For this review, use the dimensioned drawing (mm, ordinates from the lowest corner) and the shaded views. A direction names the side the tool comes from. Give positions to 0.01 mm unless a question says otherwise; leave off trailing zeros. Loops run counter-clockwise (first coordinate to the right, second up) from the corner with the lowest first, then second, coordinate; pieces in that order, holes last. Notation, with made-up numbers: (31, 52.5) -> (60, 52.5) arc R9 ccw to (60, 66.5) -> close; hole circle Ø11 at (-14, 12). An arc over 180 degrees is marked (long way). Write each question's results on one line, items separated by ' | '. Start each with the question number.
Q1. Machinability: for the marked faces 5 and 6, which of the approach directions +Z, -Z, +X, -X, +Y, -Y give a long, thin tool a straight path to every point of the face, cutting with its end or side? Answer none if there is none.
Q2. Insertion check: pin 1 Ø4 at (x, z) = (34.06, 8.38) entering from -Y; pin 2 Ø1.5 at (x, z) = (29.06, 8.38) entering from +Y. Each pin has a flat end and moves straight along its axis. Give the tip position at first contact, or say it passes through.
Q3. We need section B-B (y = 4.55). Write out the cut boundary in (x, z) (1 decimal).
Q4. Wall thickness on L1, parallel to X at y = 3.1, z = 6.5; L2, parallel to Z at x = 34, y = 2.15 (1 decimal); L3, parallel to X at y = 2.65, z = 9: over which ranges is each line inside the solid? List them lowest first. Write a range as [from, to].
Q5. Mouldability with a two-part tool opening along X and no side actions: class the marked faces 1, 2, 3 and 4 as released by +X, released by -X, zero draft, split by the parting line, or undercut.
Q6. We need section C-C (x = 9.5). Write out the cut boundary in (y, z) (1 decimal), plus the area to 3 significant figures.
Q7. We need section A-A (z = 10.5). Write out the cut boundary in (x, y), plus the area to 3 significant figures.
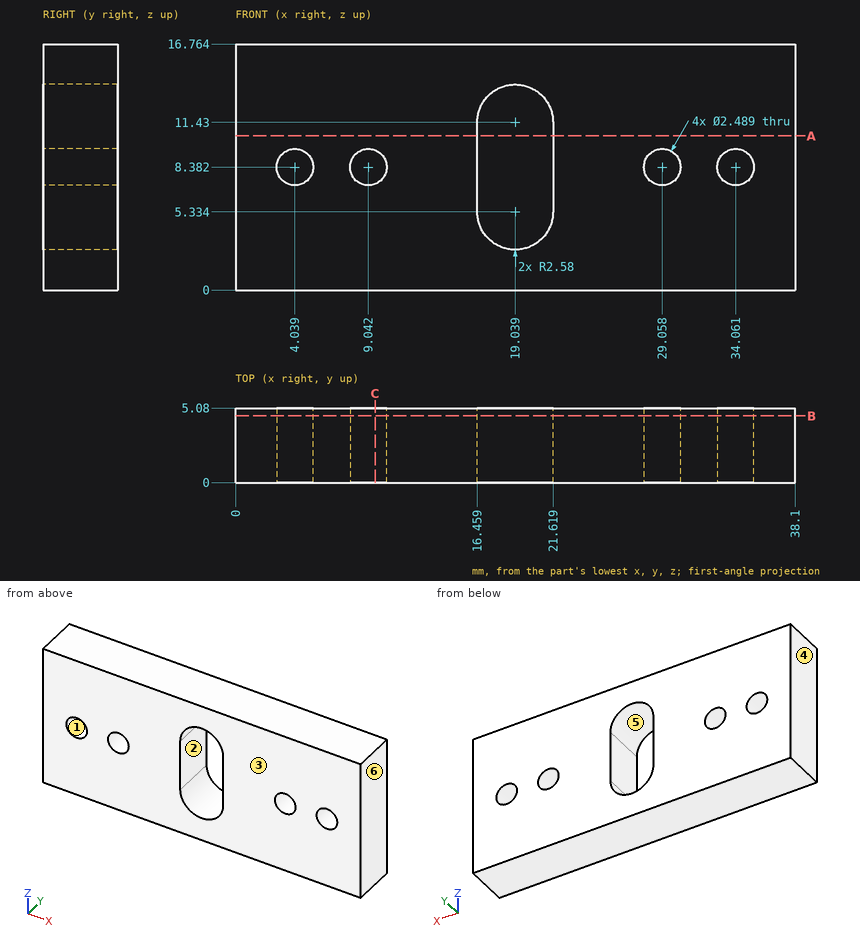
Output:
1) face 5: +Y, -Y | face 6: +Z, -Z, +X, +Y, -Y
2) pin 1: y = 0 | pin 2: through
3) outline: (0, 0) -> (38.1, 0) -> (38.1, 16.8) -> (0, 16.8) -> close; hole circle Ø2.5 at (4, 8.4); hole circle Ø2.5 at (9, 8.4); hole (16.5, 5.3) arc R2.6 ccw to (21.6, 5.3) -> (21.6, 11.4) arc R2.6 ccw to (16.5, 11.4) -> close; hole circle Ø2.5 at (29.1, 8.4); hole circle Ø2.5 at (34.1, 8.4)
4) L1: [0, 16.46], [21.62, 38.1] | L2: [0, 7.1], [9.6, 16.8] | L3: [0, 2.96], [5.12, 7.96], [10.12, 16.46], [21.62, 27.98], [30.14, 32.98], [35.14, 38.1]
5) face 1: undercut | face 2: undercut | face 3: zero draft | face 4: released by -X
6) outline: (0, 0) -> (5.1, 0) -> (5.1, 7.2) -> (0, 7.2) -> close; (0, 9.5) -> (5.1, 9.5) -> (5.1, 16.8) -> (0, 16.8) -> close | area: 73.4 mm2
7) outline: (0, 0) -> (16.46, 0) -> (16.46, 5.08) -> (0, 5.08) -> close; (21.62, 0) -> (38.1, 0) -> (38.1, 5.08) -> (21.62, 5.08) -> close | area: 167 mm2
